The model under review builds one solid part; all positions refer to its coordinate system, in mm. A direction names the side the tool comes from. Round coordinates to 2 decimals unless told otherwise and drop trailing zeros. Order: outer loops, then holes, each group sorted by start corner. A loop starts at its lowest first (then second) coordinate and runs counter-clockwise, first axis right, second up. Notation, with made-up numbers: M 56.25,-25 L 101.25,-25 A30 cw 101.25,-2 Z; hole C -36,-6 d7. An arc over 180 degrees is marked long. One line per item, written item: value. Start each with the question number.
from build123d import *
from OCP.BRepFilletAPI import BRepFilletAPI_MakeChamfer

# Parameters (mm, degrees)
BASE_DEPTH          = 10
BASE_DEPTH_BACK     = 10
ESQUISSE1_R         = 25
ESQUISSE2_R         = 25
ESQUISSE2_R_2       = 23
VIDE_GORGE_DEPTH    = 7
VIDE_JANTE_DEPTH    = 20
ESQUISSE6_R         = 3
VIDE_BLOC_AXE_DEPTH = 4
CHAN_EXT_SIZE       = 2
CHAN_EXT_SIZE_2     = 1.154700538
CHAN_INT_SIZE       = 1.154700538
CHAN_INT_SIZE_2     = 2


with BuildPart() as part:
    # Esquisse1 → BASE (new, two sides: drawn at the far end of the back side and taken through both)
    with BuildSketch(Plane(origin=(0, 0, 0), x_dir=(0, 0, -1), z_dir=(1, 0, 0)).offset(-BASE_DEPTH_BACK)):
        Circle(ESQUISSE1_R)
        with BuildLine():
            Line((-1.658312395, 2.5), (1.658312395, 2.5))
            ThreePointArc((1.658312395, 2.5), (0, -3), (-1.658312395, 2.5))
        make_face(mode=Mode.SUBTRACT)
    extrude(amount=BASE_DEPTH + BASE_DEPTH_BACK)

    # Esquisse2 → VIDE GORGE (cut)
    with BuildSketch(Plane.ZY.offset(8)):
        with Locations(Location((0, 0, 0), (0, 0, 180))):
            Circle(ESQUISSE2_R)
        Circle(ESQUISSE2_R_2, mode=Mode.SUBTRACT)
    vide_gorge = extrude(amount=-VIDE_GORGE_DEPTH, mode=Mode.SUBTRACT)

    # SYM GORGE: VIDE GORGE across plane
    add(vide_gorge.mirror(Plane(origin=(0, 0, 0), x_dir=(0, 0, 1), z_dir=(1, 0, 0))), mode=Mode.SUBTRACT)

    # Esquisse4 → VIDE JANTE (cut)
    with BuildSketch(Plane(origin=(10, 0, 0), x_dir=(0, 0, -1), z_dir=(1, 0, 0))):
        with BuildLine():
            Line((-22, 0), (-5, 0))
            ThreePointArc((-5, 0), (-4.924038765, 0.868240888), (-4.698463104, 1.710100717))
            Line((-4.698463104, 1.710100717), (-20.673237657, 7.524443153))
            ThreePointArc((-20.673237657, 7.524443153), (-21.665770566, 3.820259909), (-22, 0))
        make_face()
        with BuildLine():
            ThreePointArc((-4.698463104, -1.710100717), (-4.924038765, -0.868240888), (-5, 0))
            Line((-5, 0), (-22, 0))
            ThreePointArc((-22, 0), (-21.665770566, -3.820259909), (-20.673237657, -7.524443153))
            Line((-20.673237657, -7.524443153), (-4.698463104, -1.710100717))
        make_face()
        with BuildLine():
            Line((-13.544552457, 17.336236579), (-3.078307377, 3.940053768))
            ThreePointArc((-3.078307377, 3.940053768), (-1.545084972, 4.755282581), (0.174497484, 4.996954135))
            Line((0.174497484, 4.996954135), (0.767788927, 21.986598194))
            ThreePointArc((0.767788927, 21.986598194), (-6.798373876, 20.923243358), (-13.544552457, 17.336236579))
        make_face()
        with BuildLine():
            Line((12.302243876, 18.238826596), (2.795964517, 4.145187863))
            ThreePointArc((2.795964517, 4.145187863), (4.045084972, 2.938926261), (4.80630848, 1.378186779))
            Line((4.80630848, 1.378186779), (21.147757311, 6.064021828))
            ThreePointArc((21.147757311, 6.064021828), (17.798373876, 12.93127555), (12.302243876, 18.238826596))
        make_face()
        with BuildLine():
            ThreePointArc((4.80630848, -1.378186779), (4.045084972, -2.938926261), (2.795964517, -4.145187863))
            Line((2.795964517, -4.145187863), (12.302243876, -18.238826596))
            ThreePointArc((12.302243876, -18.238826596), (17.798373876, -12.93127555), (21.147757311, -6.064021828))
            Line((21.147757311, -6.064021828), (4.80630848, -1.378186779))
        make_face()
        with BuildLine():
            ThreePointArc((0.174497484, -4.996954135), (-1.545084972, -4.755282581), (-3.078307377, -3.940053768))
            Line((-3.078307377, -3.940053768), (-13.544552457, -17.336236579))
            ThreePointArc((-13.544552457, -17.336236579), (-6.798373876, -20.923243358), (0.767788927, -21.986598194))
            Line((0.767788927, -21.986598194), (0.174497484, -4.996954135))
        make_face()
    extrude(amount=-VIDE_JANTE_DEPTH, mode=Mode.SUBTRACT)

    # Esquisse6 → VIDE BLOC AXE (cut)
    with BuildSketch(Plane.ZY.offset(10)):
        with Locations(Location((0, 0, 0), (0, 0, 180))):
            Circle(ESQUISSE6_R)
    extrude(amount=-VIDE_BLOC_AXE_DEPTH, mode=Mode.SUBTRACT)

    # CHAN EXT
    chan_ext_edges_1 = [part.edges().sort_by_distance(p)[0] for p in [
        (-8, 0, -23),
    ]]
    chan_ext_side_1 = [part.faces().sort_by_distance(p)[0] for p in [
        (-8, 0, -23.023094011),
    ]]
    chan_ext_edges_2 = [part.edges().sort_by_distance(p)[0] for p in [
        (8, 0, -23),
    ]]
    chan_ext_side_2 = [part.faces().sort_by_distance(p)[0] for p in [
        (7.976905989, 0, -23),
    ]]
    chan_ext = BRepFilletAPI_MakeChamfer(part.part.solid().wrapped)
    for e in chan_ext_edges_1:
        chan_ext.Add(CHAN_EXT_SIZE - 0.0001, CHAN_EXT_SIZE_2 - 0.0001, e.wrapped, chan_ext_side_1[0].wrapped)
    for e in chan_ext_edges_2:
        chan_ext.Add(CHAN_EXT_SIZE_2 - 0.0001, CHAN_EXT_SIZE - 0.0001, e.wrapped, chan_ext_side_2[0].wrapped)
    add(Compound.cast(chan_ext.Shape()), mode=Mode.REPLACE)  # a hair under: the kernel refuses the full size

    # CHAN INT
    chan_int_edges_1 = [part.edges().sort_by_distance(p)[0] for p in [
        (-1, 0, -23),
    ]]
    chan_int_side_1 = [part.faces().sort_by_distance(p)[0] for p in [
        (-1.023094011, 0, -23),
    ]]
    chan_int_edges_2 = [part.edges().sort_by_distance(p)[0] for p in [
        (1, 0, -23),
    ]]
    chan_int_side_2 = [part.faces().sort_by_distance(p)[0] for p in [
        (1, 0, -23.023094011),
    ]]
    chan_int = BRepFilletAPI_MakeChamfer(part.part.solid().wrapped)
    for e in chan_int_edges_1:
        chan_int.Add(CHAN_INT_SIZE - 0.0001, CHAN_INT_SIZE_2 - 0.0001, e.wrapped, chan_int_side_1[0].wrapped)
    for e in chan_int_edges_2:
        chan_int.Add(CHAN_INT_SIZE_2 - 0.0001, CHAN_INT_SIZE - 0.0001, e.wrapped, chan_int_side_2[0].wrapped)
    add(Compound.cast(chan_int.Shape()), mode=Mode.REPLACE)  # a hair under: the kernel refuses the full size


solid = part.part
Item 1: The part is to be moulded in two halves that separate along Y. For faces 4 (the flat face through (0.14, -11.09, -7.48)), 5 (the flat face through (0.14, -10.544, 8.238)), 6 (the flat face through (-10, 0, -5)), 7 (the cylindrical face through (4.533, 22.804, -2.994)), say which applies: pulls with the +Y half, pulls with the -Y half, needs draft (parallel to the pull), parting line crosses it, or undercut.
Item 2: Clearance check with flat-ended pins moving along their axes: P1, Ø8, axis at x = 1, z = -16.5, coming from the -Y side; P2, Ø4, axis at x = 7, z = 17.5, coming from the +Y side; P3, Ø3, axis at x = 0.5, y = 10, coming from the +Z side. State where each tip first meets the part, or that it passes through.
Item 3: Wall thickness on L1, parallel to Y at x = -5.5, z = 0; L2, parallel to Z at x = 1.25, y = 0; L3, parallel to X at y = 15, z = -19: over which ranges is each line inside the solid? List them lowest first.
Item 4: Consider section C-C, the plane x = 0. Give the boundary of the cut face in (y, z), then the cut area to 3 significant figures.
Item 5: Consider section A-A, the plane x = 4.5. Give the boundary of the cut face in (y, z).
Item 6: Machinability: for faces 1 (the cylindrical face through (-4.533, 22.804, -2.994)), 2 (the flat face through (10, 0, -5)), 3 (the cylindrical face through (0.14, -4.763, 1.522)), which of the approach directions +Z, -Z, +X, -X, +Y, -Y give a long, thin tool a straight path to every point of the face, cutting with its end or side? Answer none if there is none.
Item 7: Consider section B-B, the plane y = -13. Count the separate pieces of the cut face and the enclosed holes in it, then the cut area to 3 significant figures.
Computed:
1. face 4: undercut
1. face 5: undercut
1. face 6: needs draft
1. face 7: parting line crosses it
2. P1: stops at y = -21.65
2. P2: stops at y = 19.4
2. P3: stops at z = 23.51
3. L1: y = -23 to -22, -5 to -3, 2.5 to 5, 22 to 23
3. L2: z = -24.57 to -3, 3 to 5, 22 to 24.57
3. L3: x = -10 to -7.54, -1.46 to 1.46, 7.54 to 10
4. outline: C 0,0 d50; hole M -21.99,-0.77 L -5,-0.17 A5 cw -3.94,3.08 L -17.34,13.54 A22 ccw Z; hole M -18.24,-12.3 A22 ccw -6.06,-21.15 L -1.38,-4.81 A5 cw -4.15,-2.8 Z; hole M -7.52,20.67 L -1.71,4.7 A5 cw 1.71,4.7 L 7.52,20.67 A22 ccw Z; hole M 1.38,-4.81 L 6.06,-21.15 A22 ccw 18.24,-12.3 L 4.15,-2.8 A5 cw Z; hole M 2.5,-1.66 L 2.5,1.66 A3 ccw long Z; hole M 3.94,3.08 A5 cw 5,-0.17 L 21.99,-0.77 A22 ccw 17.34,13.54 Z
4. area: 1,140 mm^2
5. outline: C 0,0 d46; hole M -21.99,-0.77 L -5,-0.17 A5 cw -3.94,3.08 L -17.34,13.54 A22 ccw Z; hole M -18.24,-12.3 A22 ccw -6.06,-21.15 L -1.38,-4.81 A5 cw -4.15,-2.8 Z; hole M -7.52,20.67 L -1.71,4.7 A5 cw 1.71,4.7 L 7.52,20.67 A22 ccw Z; hole M 1.38,-4.81 L 6.06,-21.15 A22 ccw 18.24,-12.3 L 4.15,-2.8 A5 cw Z; hole M 2.5,-1.66 L 2.5,1.66 A3 ccw long Z; hole M 3.94,3.08 A5 cw 5,-0.17 L 21.99,-0.77 A22 ccw 17.34,13.54 Z
6. face 1: none
6. face 2: +Z, -Z, +X, +Y, -Y
6. face 3: +X, -X
7. separate pieces: 3
7. enclosed holes: 0
7. area: 407 mm^2
